Geometry: final body of the model. Coordinates: model frame, mm. Face numbers are marked on the shaded views. A direction names the side the tool comes from. Give positions to 0.01 mm unless a question says otherwise; leave off trailing zeros. Order: outer loops, then holes, each group sorted by start corner. A loop starts at its lowest first (then second) coordinate and runs counter-clockwise, first axis right, second up. Notation, with made-up numbers: (-16.5, 27.5) - (-3.5, 27.5) arc R7 ccw to (-3.5, 33.5) - close; hole circle Ø4 at (15, -32). An arc over 180 degrees is marked (long way). One line per item, written item: value.
```python
from build123d import *

# Parameters (mm, degrees)
SKETCH1_R           = 7.39
SKETCH1_R_2         = 1.5
BOSS_EXTRUDE1_DEPTH = 6
BOSS_EXTRUDE2_DEPTH = 10
SKETCH2_R           = 2.65
CUT_EXTRUDE1_DEPTH  = 4.3


with BuildPart() as part:
    # Sketch1 → Boss-Extrude1 (new body)
    with BuildSketch(Plane.XY):
        Circle(SKETCH1_R)
        with Locations((0, -5)):
            Circle(SKETCH1_R_2, mode=Mode.SUBTRACT)
        with Locations((-5, 0)):
            Circle(SKETCH1_R_2, mode=Mode.SUBTRACT)
        with Locations((0, 5)):
            Circle(SKETCH1_R_2, mode=Mode.SUBTRACT)
        with BuildLine():
            ThreePointArc((1.5, 1), (0.5, 0), (1.5, -1))
            Line((1.5, -1), (5.5, -1))
            ThreePointArc((5.5, -1), (6.5, 0), (5.5, 1))
            Line((5.5, 1), (1.5, 1))
        make_face(mode=Mode.SUBTRACT)
    extrude(amount=BOSS_EXTRUDE1_DEPTH)

    # Sketch1_3 → Boss-Extrude2 (add)
    with BuildSketch(Plane.XY):
        with BuildLine():
            Line((5.5, 1), (1.5, 1))
            ThreePointArc((1.5, 1), (0.5, 0), (1.5, -1))
            Line((1.5, -1), (5.5, -1))
            ThreePointArc((5.5, -1), (6.5, 0), (5.5, 1))
        make_face()
    extrude(amount=BOSS_EXTRUDE2_DEPTH)

    # Sketch2 → Cut-Extrude1 (cut)
    with BuildSketch(Plane(origin=(0, 0, 0), x_dir=(-1, 0, 0), z_dir=(0, 0, -1))):
        Circle(SKETCH2_R)
    extrude(amount=-CUT_EXTRUDE1_DEPTH, mode=Mode.SUBTRACT)


solid = part.part
```
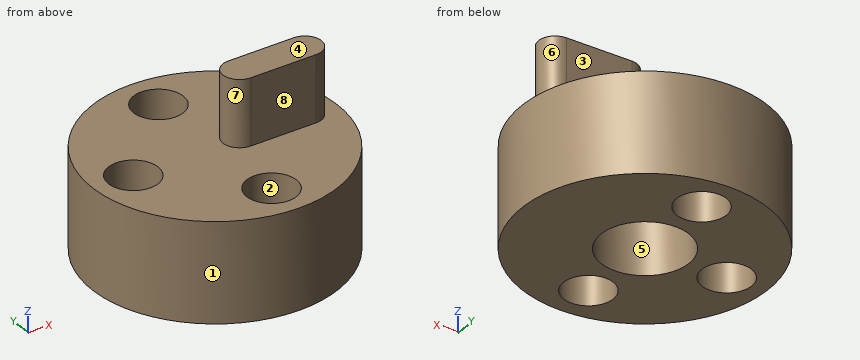
1) Section B-B, the plane x = -4. Return loops of the section in (y, z).
Answers below:
outline: (-6.21, 0) - (-1.12, 0) - (-1.12, 6) - (-6.21, 6) - close; (1.12, 0) - (6.21, 0) - (6.21, 6) - (1.12, 6) - close
2) Set-up query: the marked faces 4, 5, 6, 7 and 8. Return all of +Z, -Z, +X, -X, +Y, -Y with unobstructed straight access to the full face (end or side cutting, diameter ignored); none if empty.
Answers below:
face 4: +Z, +X, -X, +Y, -Y
face 5: -Z
face 6: +Z, +X
face 7: +Z, -X
face 8: +Z, +X, -X, -Y
3) Material intervals for line 1 along Y through (x, z) = (0, 3.3); line 2 along Z through (x, y) = (-5.5, -1.75); line 3 along X through (y, z) = (5.5, 4.5), sorted ascending.
Answers below:
line 1: -7.39 to -6.5, -3.5 to -2.65, 2.65 to 3.5, 6.5 to 7.39
line 2: 0 to 6
line 3: -4.94 to -1.41, 1.41 to 4.94
4) Section D-D, the plane z = 7. Return loops of the section in (x, y), then the cut area to 3 significant figures.
Answers below:
outline: (1.5, -1) - (5.5, -1) arc R1 ccw to (5.5, 1) - (1.5, 1) arc R1 ccw to start
area: 11.1 mm^2
5) Mould query, pull axis X, two halves, no side actions, for the marked faces 1, 2 and 3. Classes: released by +X, released by -X, zero draft, split by the parting line, or undercut.
Answers below:
face 1: split by the parting line
face 2: undercut
face 3: zero draft
6) First-contact query: pin 1 (3 mm diameter, centred on x = 0, y = 0, fed in from +Z); pin 2 (3 mm diameter, centred on x = 4, z = 8.5, fed in from +Y); pin 3 (4 mm diameter, centred on y = -4, z = 5, fed in from -X); pin 4 (5 mm diameter, centred on x = -5, y = 0, fed in from +Z). Flat tips, straight axial feed; report the tip coordinate or a pass-through.
Answers below:
pin 1: z = 10
pin 2: y = 1
pin 3: x = -7.11
pin 4: z = 6
7) Section C-C, the plane x = -1. Return loops of the section in (y, z).
Answers below:
outline: (-7.32, 0) - (-6.12, 0) - (-6.12, 6) - (-7.32, 6) - close; (-3.88, 0) - (-2.45, 0) - (-2.45, 4.3) - (2.45, 4.3) - (2.45, 0) - (3.88, 0) - (3.88, 6) - (-3.88, 6) - close; (6.12, 0) - (7.32, 0) - (7.32, 6) - (6.12, 6) - close
8) Section A-A, the plane y = 0.5. Return loops of the section in (x, z), then the cut area to 3 significant figures.
Answers below:
outline: (-7.37, 0) - (-6.41, 0) - (-6.41, 6) - (-7.37, 6) - close; (-3.59, 0) - (-2.6, 0) - (-2.6, 4.3) - (2.6, 4.3) - (2.6, 0) - (7.37, 0) - (7.37, 6) - (6.37, 6) - (6.37, 10) - (0.63, 10) - (0.63, 6) - (-3.59, 6) - close
area: 72.1 mm^2
